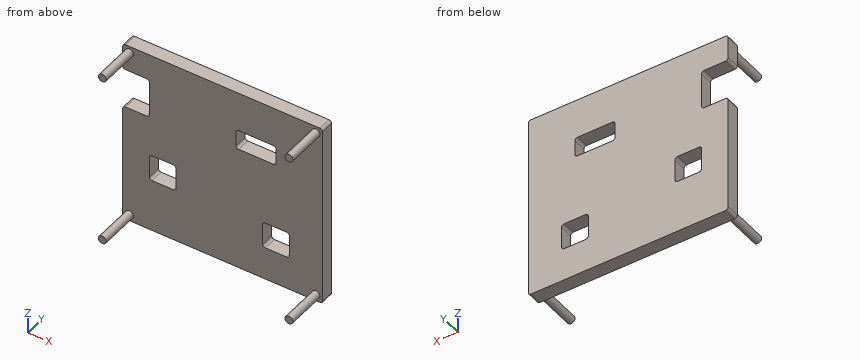
```python
from build123d import *

# Parameters (mm, degrees)
SKETCH1_W           = 150
SKETCH1_H           = 140
BOSS_EXTRUDE1_DEPTH = 10
SKETCH2_R           = 3
BOSS_EXTRUDE2_DEPTH = 30
SKETCH4_W           = 20
SKETCH4_H           = 20
CUT_EXTRUDE2_DEPTH  = 111.113577728
SKETCH6_W           = 20
SKETCH6_H           = 30
CUT_EXTRUDE3_DEPTH  = 111.113577728
SKETCH7_W           = 30
SKETCH7_H           = 15
CUT_EXTRUDE4_DEPTH  = 111.113577728
SKETCH8_W           = 20
SKETCH8_H           = 20
CUT_EXTRUDE5_DEPTH  = 111.113577728
FILLET2_R           = 2


with BuildPart() as part:
    # Sketch1 → Boss-Extrude1 (new body)
    with BuildSketch(Plane(origin=(0, 0, 0), x_dir=(1, 0, 0), z_dir=(0, 1, 0))):
        Rectangle(SKETCH1_W, SKETCH1_H)
    extrude(amount=BOSS_EXTRUDE1_DEPTH)

    # Sketch2 → Boss-Extrude2 (add)
    with BuildSketch(Plane.XZ):
        with Locations(Location((-70, 65, 0), (0, 0, 90))):
            Circle(SKETCH2_R)
        with Locations(Location((70, 65, 0), (0, 0, 90))):
            Circle(SKETCH2_R)
        with Locations(Location((70, -65, 0), (0, 0, 90))):
            Circle(SKETCH2_R)
        with Locations(Location((-70, -65, 0), (0, 0, 90))):
            Circle(SKETCH2_R)
    extrude(amount=BOSS_EXTRUDE2_DEPTH)

    # Sketch4 → Cut-Extrude2 (cut, through all)
    with BuildSketch(Plane(origin=(0, 10, 0), x_dir=(1, 0, 0), z_dir=(0, 1, 0))):
        with Locations((-45, 20)):
            Rectangle(SKETCH4_W, SKETCH4_H)
    extrude(amount=-CUT_EXTRUDE2_DEPTH, mode=Mode.SUBTRACT)

    # Sketch6 → Cut-Extrude3 (cut, through all)
    with BuildSketch(Plane(origin=(0, 10, 0), x_dir=(1, 0, 0), z_dir=(0, 1, 0))):
        with Locations((-65, -35)):
            Rectangle(SKETCH6_W, SKETCH6_H)
    extrude(amount=-CUT_EXTRUDE3_DEPTH, mode=Mode.SUBTRACT)

    # Sketch7 → Cut-Extrude4 (cut, through all)
    with BuildSketch(Plane(origin=(0, 10, 0), x_dir=(1, 0, 0), z_dir=(0, 1, 0))):
        with Locations((25, -32.5)):
            Rectangle(SKETCH7_W, SKETCH7_H)
    extrude(amount=-CUT_EXTRUDE4_DEPTH, mode=Mode.SUBTRACT)

    # Sketch8 → Cut-Extrude5 (cut, through all)
    with BuildSketch(Plane(origin=(0, 10, 0), x_dir=(1, 0, 0), z_dir=(0, 1, 0))):
        with Locations((40, 35)):
            Rectangle(SKETCH8_W, SKETCH8_H)
    extrude(amount=-CUT_EXTRUDE5_DEPTH, mode=Mode.SUBTRACT)

    # Fillet2
    fillet2_edges = [part.edges().sort_by_distance(p)[0] for p in [
        (-35, 5, -30),
        (-35, 5, -10),
        (-55, 5, -10),
        (-55, 5, -30),
        (-75, 5, 50),
        (-75, 5, 20),
        (-55, 5, 20),
        (-55, 5, 50),
        (40, 5, 25),
        (40, 5, 40),
        (10, 5, 40),
        (10, 5, 25),
        (-75, 5, -70),
        (75, 5, -70),
        (75, 5, 70),
        (-75, 5, 70),
        (30, 5, -25),
        (30, 5, -45),
        (50, 5, -45),
        (50, 5, -25),
    ]]
    fillet(fillet2_edges, radius=FILLET2_R)


solid = part.part
```
CAD build for the part. Positions are in the model's coordinates, mm. Coordinates: 2 decimals unless noted, no trailing zeros. Order: outer loops, then holes, each group sorted by start corner. A loop starts at its lowest first (then second) coordinate and runs counter-clockwise, first axis right, second up. Notation, with made-up numbers: (77, 77.25) - (84, 77.25) arc R13 cw to (84, 102.25) - close; hole circle Ø9 at (13.5, 89). An arc over 180 degrees is marked (long way). Use a Markdown table: item, result. Add a question column.
(1) Saw through at C-C (z = 65). Give the cut face in (x, y), then the cut area to 3 significant figures.
(2) Drill centre lines: line 1 along Z through (x, y) = (-47, 5.5); line 2 along Y through (x, z) = (-44, 50). Where is each one in solid material? Low to high. Write a range as [from, to].
(3) Saw through at B-B (x = -47.5). Give the cut face in (y, z), then the cut area to 3 significant figures.
(4) Flat gauge pins, fed straight in: pin 1 (12 mm diameter, centred on x = -50, z = 50, fed in from -Y); pin 2 (8 mm diameter, centred on y = 6, z = 33.5, fed in from -X). Where does each tip first touch, or does it go through?
(5) Saw through at A-A (z = -40). Give the cut face in (x, y), then the cut area to 3 significant figures.
(6) Saw through at D-D (x = -70). Give the cut face in (y, z).
Solved:
| question | item | result |
|---|---|---|
| 1 | outline | (-75, 0) - (-73, 0) - (-73, -30) - (-67, -30) - (-67, 0) - (67, 0) - (67, -30) - (73, -30) - (73, 0) - (75, 0) - (75, 10) - (-75, 10) - close |
| 1 | area | 1,860 mm² |
| 2 | line 1 | z = [-70, -30], [-10, 70] |
| 2 | line 2 | y = [0, 10] |
| 3 | outline | (0, -70) - (10, -70) - (10, -30) - (0, -30) - close; (0, -10) - (10, -10) - (10, 70) - (0, 70) - close |
| 3 | area | 1,200 mm² |
| 4 | pin 1 | stops at y = 0 |
| 4 | pin 2 | stops at x = -55 |
| 5 | outline | (-75, 0) - (30, 0) - (30, 10) - (-75, 10) - close; (50, 0) - (75, 0) - (75, 10) - (50, 10) - close |
| 5 | area | 1,300 mm² |
| 6 | outline | (-30, -68) - (0, -68) - (0, -70) - (10, -70) - (10, 20) - (0, 20) - (0, -62) - (-30, -62) - close; (-30, 62) - (0, 62) - (0, 50) - (10, 50) - (10, 70) - (0, 70) - (0, 68) - (-30, 68) - close |
